Source: three-view drawing plus pictorial views. Frame: mm from the lowest corner of the part. A direction names the side the tool comes from. Give positions to 0.01 mm unless a question says otherwise; leave off trailing zeros. Order: outer loops, then holes, each group sorted by start corner. A loop starts at its lowest first (then second) coordinate and runs counter-clockwise, first axis right, second up. Notation, with made-up numbers: M -18.75,-19 L 32.25,-19 A22 ccw 32.25,16 Z; hole C -39,33 d9. An arc over 180 degrees is marked long. Use CSV: the item, a comma, the result in double quotes. Start each with the question number.
1. Section query B-B, the plane x = 23.5. Return the cut outline in (y, z) (3 decimals), plus the area to 3 significant figures.
2. Line query: line 1 along X through (y, z) = (2.5, 4.75); line 2 along X through (y, z) = (8.75, 3.75); line 3 along Y through (x, z) = (13.5, 3.5). Output: solid intervals per line, ascending. Write a range as [from, to].
3. Section query C-C, the plane z = 1. Return the cut outline in (x, y).
4. Mould query, pull axis Z, two halves, no side actions, for the marked faces 1, 2, 3 and 4. Classes: released by +Z, released by -Z, zero draft, split by the parting line, or undercut.
5. Section query A-A, the plane y = 8.75. Return the cut outline in (x, z) (3 decimals), plus the area to 3 significant figures.
6. Reachability of the marked faces 5 and 6 from +Z, -Z, +X, -X, +Y, -Y: full face, straight path, thin tool, end or side. Return the list, or none.
7. Pin query (flat end, axial travel): P1, Ø3.5, axis at x = 23.5, z = 3.375, coming from the +Y side; P2, Ø5, axis at x = 11.5, y = 8, coming from the -Z side. Return the tip coordinate at first contact, or that it passes through.
8. Section query D-D, the plane y = 5.5. Return the cut outline in (x, z) (3 decimals), plus the area to 3 significant figures.
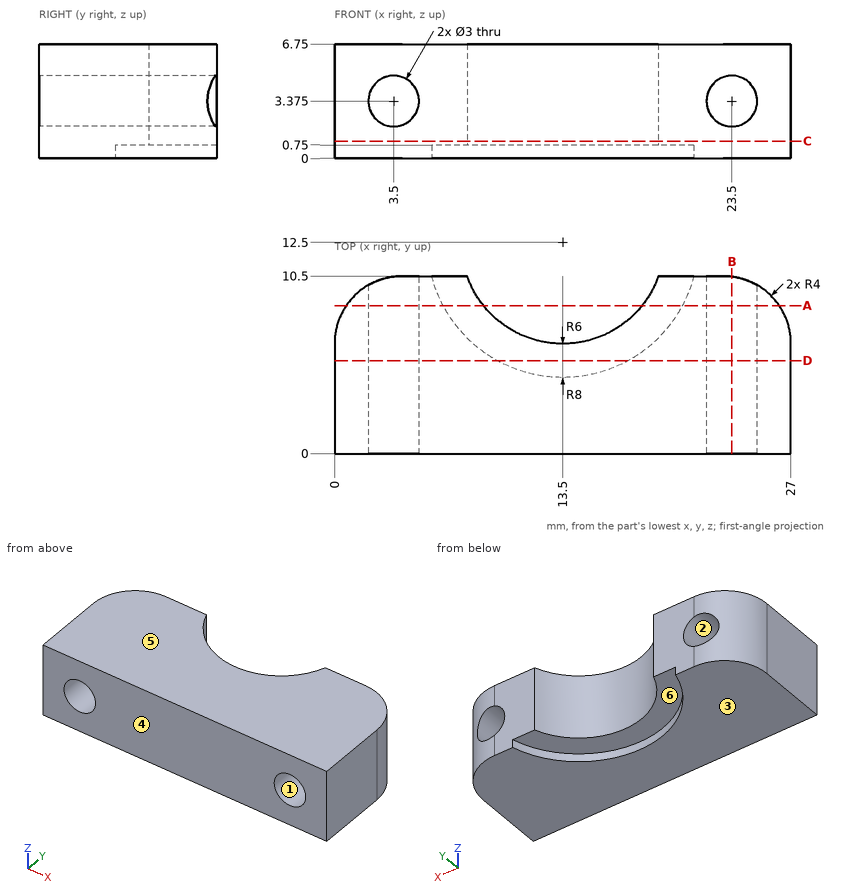
Result set:
1,outline,"M 0,0 L 10.469,0 L 10.469,1.875 L 0,1.875 Z; M 0,4.875 L 10.469,4.875 L 10.469,6.75 L 0,6.75 Z"
1,area,"39.3 mm2"
2,line 1,"[0, 2.9], [4.1, 22.9], [24.1, 27]"
2,line 2,"[0.69, 2.05], [4.95, 8.82], [18.18, 22.05], [24.95, 26.31]"
2,line 3,"[0, 6.5]"
3,outline,"M 0,0 L 27,0 L 27,6.5 A4 ccw 23,10.5 L 19.16,10.5 A6 cw 7.84,10.5 L 4,10.5 A4 ccw 0,6.5 Z"
4,face 1,"undercut"
4,face 2,"undercut"
4,face 3,"released by -Z"
4,face 4,"zero draft"
5,outline,"M 0.693,0 L 6.433,0 L 6.433,0.75 L 8.816,0.75 L 8.816,6.75 L 0.693,6.75 Z; M 18.184,0.75 L 20.567,0.75 L 20.567,0 L 26.307,0 L 26.307,6.75 L 18.184,6.75 Z; hole C 3.5,3.375 d3; hole C 23.5,3.375 d3"
5,area,"92.0 mm2"
6,face 5,"+Z, +X, -X, +Y, -Y"
6,face 6,"-Z, +Y"
7,P1,"y = 10.5"
7,P2,"z = 0.75"
8,outline,"M 0,0 L 9.627,0 L 9.627,0.75 L 17.373,0.75 L 17.373,0 L 27,0 L 27,6.75 L 0,6.75 Z; hole C 3.5,3.375 d3; hole C 23.5,3.375 d3"
8,area,"162 mm2"
